The model under review builds one solid part; all positions refer to its coordinate system, in mm. A direction names the side the tool comes from. Coordinates: 2 decimals unless noted, no trailing zeros. Order: outer loops, then holes, each group sorted by start corner. A loop starts at its lowest first (then second) coordinate and runs counter-clockwise, first axis right, second up. Notation, with made-up numbers: M -2.75,11 L 54.25,11 A30 ccw 54.25,41 Z; hole C 22,-11 d2. An arc over 180 degrees is marked long. One line per item, written item: value.
```python
from build123d import *

# Parameters (mm, degrees)
F0_W     = 60.706
F0_H     = 35.052
F1_DEPTH = 12.7
F2_T     = -1.5875
F3_R     = 2.54


with BuildPart() as f1:
    # F0 (on Top) → F1 (new body)
    with BuildSketch(Plane.XY):
        Rectangle(F0_W, F0_H)
    extrude(amount=F1_DEPTH)

    # F2
    f2_openings = [f1.faces().sort_by_distance(p)[0] for p in [
        (0, 0, 12.7),
    ]]
    offset(amount=F2_T, openings=f2_openings)

    # F3
    f3_edges = [f1.edges().sort_by_distance(p)[0] for p in [
        (-30.353, -17.526, 6.35),
        (-30.353, 17.526, 6.35),
        (30.353, -17.526, 6.35),
        (30.353, 17.526, 6.35),
    ]]
    fillet(f3_edges, radius=F3_R)


solid = f1.part
```
(1) Tool access review of faces 5 (the flat face through (-30.353, 0, 6)), 6 (the flat face through (0, 0, 1.588)): name each direction out of +Z, -Z, +X, -X, +Y, -Y from which nothing blocks a thin tool from reaching the whole face with its end or side.
Geometry results:
face 5: +Z, -Z, -X, +Y, -Y
face 6: +Z
(2) We need section C-C, the plane y = -12.5. State the section outline as (x, z) points.
Geometry results:
outline: M -30.35,0 L 30.35,0 L 30.35,12.7 L 28.77,12.7 L 28.77,1.59 L -28.77,1.59 L -28.77,12.7 L -30.35,12.7 Z
(3) We need section B-B, the plane x = 1.5. State the section outline as (y, z) points, plus the area to 3 significant figures.
Geometry results:
outline: M -17.53,0 L 17.53,0 L 17.53,12.7 L 15.94,12.7 L 15.94,1.59 L -15.94,1.59 L -15.94,12.7 L -17.53,12.7 Z
area: 90.9 mm2
(4) Insertion check: pin 1 Ø16 at (x, y) = (4, 7) entering from +Z. The pin has a flat end and moves straight along its axis. Give the tip position at first contact, or say it passes through.
Geometry results:
pin 1: stops at z = 1.59
(5) Mouldability with a two-part tool opening along X and no side actions: class faces 1 (the cylindrical face through (29.63, 16.76, 6.44)), 2 (the cylindrical face through (-29.63, 16.76, 6.44)), 3 (the flat face through (0, 15.938, 7)), 4 (the flat face through (28.766, 0, 7)) as +X half, -X half, draft (parallel to the pull), parting line (faces both ways), or undercut.
Geometry results:
face 1: +X half
face 2: -X half
face 3: undercut
face 4: undercut
(6) For L1, parallel to X at y = 1, z = 4.25; L2, parallel to Y at x = 17, z = 10; L3, parallel to Z at x = -25.5, y = 13, list the stretches that pass through material, from the lowest coordinate up.
Geometry results:
L1: x = -30.35 to -28.77, 28.77 to 30.35
L2: y = -17.53 to -15.94, 15.94 to 17.53
L3: z = 0 to 1.59
(7) We need section A-A, the plane z = 3. State the section outline as (x, y) points.
Geometry results:
outline: M -30.35,-14.99 A2.54 ccw -27.81,-17.53 L 27.81,-17.53 A2.54 ccw 30.35,-14.99 L 30.35,14.99 A2.54 ccw 27.81,17.53 L -27.81,17.53 A2.54 ccw -30.35,14.99 Z; hole M -28.77,-15.94 L 28.77,-15.94 L 28.77,15.94 L -28.77,15.94 Z
